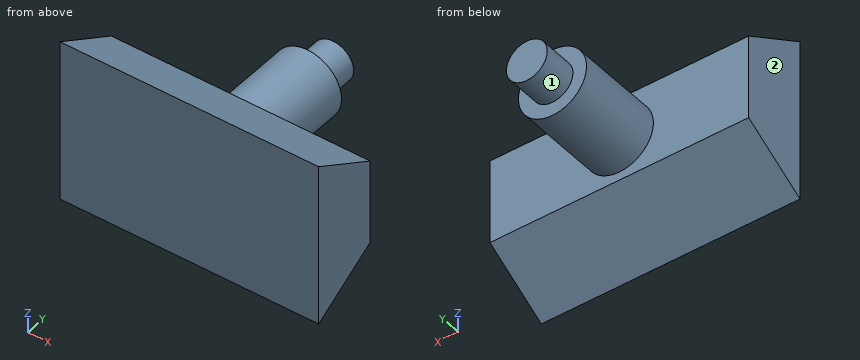
Autodesk Inventor part; units mm, degrees
ref_plane "YZ Plane" through (0, 0, 0) normal (1, 0, 0) x (0, 1, 0)
ref_plane "XZ Plane" through (0, 0, 0) normal (0, 1, 0) x (-1, 0, 0)
ref_plane "XY Plane" through (0, 0, 0) normal (0, 0, 1) x (1, 0, 0)
sketch "Sketch4" plane through (0, 0, 0) normal (1, 0, 0) x (0, 1, 0)
  line L0 (0, 0) -> (0, -12)
  line L1 (0, -12) -> (10, -6.2265)
  line L2 (10, -6.2265) -> (10, 6.2265)
  line L3 (10, 6.2265) -> (0, 12)
  line L4 (0, 12) -> (0, 0)
  line L5 (0, 0) -> (10, 0)
  dimension "d31" = 60
  dimension "d32" = 60
  dimension "d33" = 10
  dimension "d34" = 12
extrude "Extrusion3" add sketch "Sketch4" along normal mid plane 38
sketch "Sketch5" plane through (-19, 10, 6.2265) normal (0, 1, 0) x (1, 0, 0)
  circle A0 centre (19, 6.2265) radius 5
  dimension "d37" = 10
extrude "Extrusion4" add sketch "Sketch5" along normal blind 13
sketch "Sketch6" plane through (0, 23, 0) normal (0, 1, 0) x (1, 0, 0)
  circle A0 centre (0, 0) radius 3
  point P0 (0, 0)
  dimension "d40" = 6
extrude "Extrusion5" add sketch "Sketch6" along normal blind 5
properties part number "Sketch" material "Acero inoxidable, austenítico"
Verification items for the finished model (mm, model axes). Face numbers are marked on the shaded views. A direction names the side the tool comes from. Round coordinates to 2 decimals unless told otherwise and drop trailing zeros. Write each loop counter-clockwise with the first axis right and the second up, starting at its lowest first coordinate (ties: lowest second). Pieces come first, ordered by that corner, then holes. Notation, with made-up numbers: (-22, 5.25) -> (3, 5.25) arc R14 ccw to (3, 14.25) -> close; hole circle Ø6 at (16.25, 85.5). An arc over 180 degrees is marked (long way). Write each question's results on one line, items separated by ' | '.
Q1. Sectioned sample at C-C, the plane y = 19. Record the boundary of the cut face in (x, z), and give its area (3 significant figures).
Derived:
outline: circle Ø10 at (0, 0) | area: 78.5 mm²
Q2. Sectioned sample at D-D, the plane z = -4. Record the boundary of the cut face in (x, y), and give its area (3 significant figures).
Derived:
outline: (-19, 0) -> (19, 0) -> (19, 10) -> (3, 10) -> (3, 23) -> (-3, 23) -> (-3, 10) -> (-19, 10) -> close | area: 458 mm²
Q3. Sectioned sample at A-A, the plane z = 0. Record the boundary of the cut face in (x, y).
Derived:
outline: (-19, 0) -> (19, 0) -> (19, 10) -> (5, 10) -> (5, 23) -> (3, 23) -> (3, 28) -> (-3, 28) -> (-3, 23) -> (-5, 23) -> (-5, 10) -> (-19, 10) -> close
Q4. Go/stop test with flat-tipped pins: pin 1 Ø10 at (y, z) = (20.5, -7) entering from +X; pin 2 Ø12 at (x, z) = (-14, -8) entering from +Y; pin 3 Ø8 at (y, z) = (17, 4.5) entering from +X; pin 4 Ø1.5 at (x, z) = (-5.5, 0) entering from -Y. Record where each tip stops, or that it passes through.
Derived:
pin 1: stops at x = 4.58 | pin 2: stops at y = 10 | pin 3: stops at x = 4.97 | pin 4: stops at y = 0
Q5. Sectioned sample at B-B, the plane x = 0. Record the boundary of the cut face in (y, z), and give its area (3 significant figures).
Derived:
outline: (0, -12) -> (10, -6.23) -> (10, -5) -> (23, -5) -> (23, -3) -> (28, -3) -> (28, 3) -> (23, 3) -> (23, 5) -> (10, 5) -> (10, 6.23) -> (0, 12) -> close | area: 342 mm²
Q6. Thickness scan on probe 1 along Z at (x, y) = (4, 18.25); probe 2 along Y at (x, z) = (-5.5, 2.5); probe 3 along X at (y, z) = (21.25, 2.5). Record the ranges inside material, lowest first.
Derived:
probe 1: z = -3 to 3 | probe 2: y = 0 to 10 | probe 3: x = -4.33 to 4.33
Q7. Access from +Z, -Z, +X, -X, +Y, -Y to the whole of each face (thin tool, end or side, straight path). Record for the marked faces 1 and 2.
Derived:
face 1: +Y | face 2: +Z, -Z, -X, +Y, -Y
